Autodesk Inventor part; units mm, degrees
ref_plane "YZ Plane" through (0, 0, 0) normal (1, 0, 0) x (0, 1, 0)
ref_plane "XZ Plane" through (0, 0, 0) normal (0, 1, 0) x (-1, 0, 0)
ref_plane "XY Plane" through (0, 0, 0) normal (0, 0, 1) x (1, 0, 0)
sketch "Sketch1" plane through (0, 0, 0) normal (0, 0, 1) x (1, 0, 0)
  line L0 (0, 0) -> (7.62, 0)
  line L1 (7.62, 0) -> (7.62, 2.5)
  line L2 (7.62, 2.5) -> (0, 2.5)
  line L3 (0, 2.5) -> (0, 0)
  dimension "d0" = 7.62
  dimension "d1" = 2.5
extrude "Extrusion1" add sketch "Sketch1" along normal blind 2.54
sketch "Sketch2" plane through (0, 0, 2.54) normal (0, 0, 1) x (1, 0, 0)
  line L0 (0.95, 1.57) -> (1.59, 1.57)
  line L1 (1.59, 1.57) -> (1.59, 0.93)
  line L2 (1.59, 0.93) -> (0.95, 0.93)
  line L3 (0.95, 0.93) -> (0.95, 1.57)
  line L4 (3.49, 1.57) -> (4.13, 1.57)
  line L5 (4.13, 1.57) -> (4.13, 0.93)
  line L6 (4.13, 0.93) -> (3.49, 0.93)
  line L7 (3.49, 0.93) -> (3.49, 1.57)
  line L8 (6.03, 1.57) -> (6.67, 1.57)
  line L9 (6.67, 1.57) -> (6.67, 0.93)
  line L10 (6.67, 0.93) -> (6.03, 0.93)
  line L11 (6.03, 0.93) -> (6.03, 1.57)
  line L12 (7.62, 2.5) -> (0, 2.5)
  line L13 (0, 2.5) -> (0, 0)
  dimension "d4" = 0.64
  dimension "d5" = 0.64
  dimension "d6" = 0.64
  dimension "d7" = 0.64
  dimension "d8" = 2.54
  dimension "d9" = 2.54
  dimension "d10" = 0.93
  dimension "d11" = 0.95
extrude "Extrusion2" add sketch "Sketch2" along normal blind 3
sketch "Sketch3" plane through (0, 0, 0) normal (0, 0, -1) x (-1, 0, 0)
  line L0 (-6.03, 0.93) -> (-6.67, 0.93)
  line L1 (-6.67, 0.93) -> (-6.67, 1.57)
  line L2 (-6.67, 1.57) -> (-6.03, 1.57)
  line L3 (-6.03, 1.57) -> (-6.03, 0.93)
  line L4 (-3.49, 0.93) -> (-4.13, 0.93)
  line L5 (-4.13, 0.93) -> (-4.13, 1.57)
  line L6 (-4.13, 1.57) -> (-3.49, 1.57)
  line L7 (-3.49, 1.57) -> (-3.49, 0.93)
  line L8 (-0.95, 0.93) -> (-1.59, 0.93)
  line L9 (-1.59, 0.93) -> (-1.59, 1.57)
  line L10 (-1.59, 1.57) -> (-0.95, 1.57)
  line L11 (-0.95, 1.57) -> (-0.95, 0.93)
  point P0 (0, 0)
extrude "Extrusion3" add sketch "Sketch3" along normal blind 6
chamfer "Chamfer1" distance 0.2 angle 45 24 edges at (1.27, 1.57, -6) (1.59, 1.25, -6) (1.27, 0.93, -6) (0.95, 1.25, -6) (3.81, 1.57, -6) (4.13, 1.25, -6) (3.81, 0.93, -6) (3.49, 1.25, -6) (6.03, 1.25, -6) (6.35, 1.57, -6) (6.67, 1.25, -6) (6.35, 0.93, -6) (6.67, 1.25, 5.54) (6.35, 1.57, 5.54) (6.03, 1.25, 5.54) (6.35, 0.93, 5.54) (4.13, 1.25, 5.54) (3.81, 0.93, 5.54) (3.49, 1.25, 5.54) (3.81, 1.57, 5.54) (1.59, 1.25, 5.54) (1.27, 0.93, 5.54) (0.95, 1.25, 5.54) (1.27, 1.57, 5.54)
sketch "Sketch4" plane through (0, 0, 2.54) normal (0, 0, 1) x (1, 0, 0)
  circle A0 centre (6.35, 1.25) radius 0.5
  circle A1 centre (1.27, 1.25) radius 0.5
  line L0 (0, 2.5) -> (0, 0)
  line L1 (0, 0) -> (7.62, 0)
  line L2 (7.62, 0) -> (7.62, 2.5)
  dimension "d21" = 1
  dimension "d22" = 1.27
  dimension "d23" = 1.25
  dimension "d24" = 1.25
  dimension "d25" = 1.27
extrude "Extrusion4" add sketch "Sketch4" along normal blind 0.1
equation "\"d5\" = d4"
equation "\"d6\" = d4"
equation "\"d7\" = d4"
equation "\"d9\" = d8"
equation "\"d24\" = d23"
equation "\"d25\" = d22"
properties part number "Male_Pin_1x3"
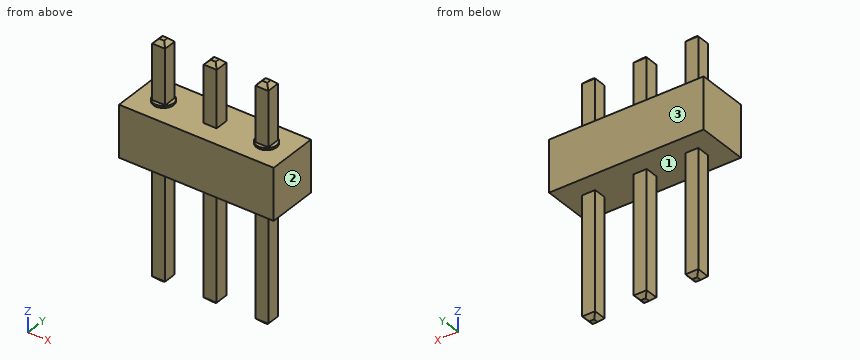
Geometry: final body of the model. Coordinates: model frame, mm. Face numbers are marked on the shaded views. Round coordinates to 2 decimals unless told otherwise and drop trailing zeros. Write each loop counter-clockwise with the first axis right and the second up, starting at its lowest first coordinate (ties: lowest second). Pieces come first, ordered by that corner, then holes. Notation, with made-up numbers: M 89,-38 L 121,-38 A24 cw 121,-4 Z; hole C 26,56.5 d8. An arc over 180 degrees is marked long. Write item = value, one per line.
Item 1: Section query C-C on y = 0.6. Return loops of the section in (x, z), then the cut area to 3 significant figures.
Findings:
outline = M 0,0 L 7.62,0 L 7.62,2.54 L 0,2.54 Z
area = 19.4 mm^2
Item 2: Material intervals for line 1 along X through (y, z) = (1.4, 4); line 2 along Z through (x, y) = (0.5, 1.65); line 3 along Y through (x, z) = (1.25, -3.5), sorted ascending. Write a range as [from, to].
Findings:
line_1 = [0.95, 1.59], [3.49, 4.13], [6.03, 6.67]
line_2 = [0, 2.54]
line_3 = [0.93, 1.57]
Item 3: Pin query (flat end, axial travel): P1, Ø0.7, axis at y = 1.5, z = 3.5, coming from the -X side; P2, Ø0.7, axis at x = 1, z = 3.5, coming from the +Y side; P3, Ø0.5, axis at x = 1, z = -1.5, coming from the -Y side. Return the tip coordinate at first contact, or that it passes through.
Findings:
P1 = 0.95
P2 = 1.57
P3 = 0.93
Item 4: Pull-direction query (X, two-part tool) for the marked faces 1, 2 and 3; classes: pulls with the +X half, pulls with the -X half, needs draft (parallel to the pull), parting line crosses it, or undercut.
Findings:
face_1 = undercut
face_2 = pulls with the +X half
face_3 = needs draft
Item 5: Section query B-B on x = 1.27. Return loops of the section in (y, z), then the cut area to 3 significant figures.
Findings:
outline = M 0,0 L 0.93,0 L 0.93,-5.8 L 1.13,-6 L 1.37,-6 L 1.57,-5.8 L 1.57,0 L 2.5,0 L 2.5,2.54 L 1.75,2.54 L 1.75,2.64 L 1.57,2.64 L 1.57,5.34 L 1.37,5.54 L 1.13,5.54 L 0.93,5.34 L 0.93,2.64 L 0.75,2.64 L 0.75,2.54 L 0,2.54 Z
area = 12.1 mm^2
Item 6: Section query A-A on z = -4. Return loops of the section in (x, y), then the cut area to 3 significant figures.
Findings:
outline = M 0.95,0.93 L 1.59,0.93 L 1.59,1.57 L 0.95,1.57 Z; M 3.49,0.93 L 4.13,0.93 L 4.13,1.57 L 3.49,1.57 Z; M 6.03,0.93 L 6.67,0.93 L 6.67,1.57 L 6.03,1.57 Z
area = 1.23 mm^2
Item 7: Section query D-D on x = 4.5. Return loops of the section in (y, z), then the cut area to 3 significant figures.
Findings:
outline = M 0,0 L 2.5,0 L 2.5,2.54 L 0,2.54 Z
area = 6.35 mm^2
